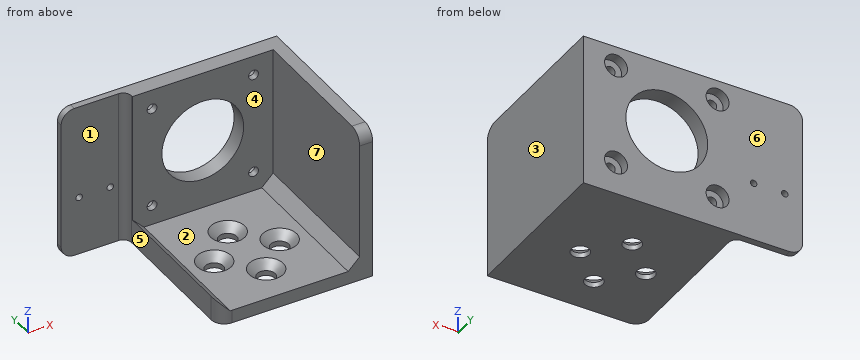
from build123d import *

# Parameters (mm, degrees)
SKETCH_2_W                  = 47
SKETCH_2_H                  = 47
EXTRUDE_1_DEPTH             = 4
SKETCH_3_W                  = 47
SKETCH_3_H                  = 2
EXTRUDE_2_DEPTH             = 43
SKETCH_4_W                  = 4
SKETCH_4_H                  = 45
EXTRUDE_3_DEPTH             = 43
SKETCH_5_R                  = 12.5
CUT_EXTRUDE_1_DEPTH         = 81.268300094
M3X0_5_2_D                  = 3
HOLE_WIZARD_M5_1_AT_2_COUNT = 2
HOLE_WIZARD_M5_1_AT_2_PITCH = 14.142135624
HOLE_WIZARD_M5_1_AT_3_COUNT = 2
HOLE_WIZARD_M5_1_AT_3_PITCH = 20
HOLE_WIZARD_M5_1_AT_4_COUNT = 2
HOLE_WIZARD_M5_1_AT_4_PITCH = 14.142135624
EXTRUDE_6_DEPTH             = 45
EXTRUDE_7_DEPTH             = 45
SKETCH_23_W                 = 67
SKETCH_23_H                 = 47
SKETCH_23_R                 = 3.5
SKETCH_23_R_2               = 12.5
EXTRUDE_10_DEPTH            = 3
M2X0_4_1_D                  = 2
SKETCH_27_W                 = 47
SKETCH_27_H                 = 1
CUT_EXTRUDE_2_DEPTH         = 20
FILLET_1_R                  = 2.5
FILLET_2_R                  = 4


with BuildPart() as part:
    # ｽｹｯﾁ2 → ﾎﾞｽ - 押し出し1 (new body)
    with BuildSketch(Plane.XY):
        with Locations((23.5, 23.5)):
            Rectangle(SKETCH_2_W, SKETCH_2_H)
    extrude(amount=EXTRUDE_1_DEPTH)

    # ｽｹｯﾁ3 → ﾎﾞｽ - 押し出し2 (add)
    with BuildSketch(Plane.XY.offset(4)):
        with Locations((23.5, 46)):
            Rectangle(SKETCH_3_W, SKETCH_3_H)
    extrude(amount=EXTRUDE_2_DEPTH)

    # ｽｹｯﾁ4 → ﾎﾞｽ - 押し出し3 (add)
    with BuildSketch(Plane.XY.offset(4)):
        with Locations((45, 22.5)):
            Rectangle(SKETCH_4_W, SKETCH_4_H)
    extrude(amount=EXTRUDE_3_DEPTH)

    # ｽｹｯﾁ5 → ｶｯﾄ - 押し出し1 (cut, through all)
    with BuildSketch(Plane.XZ.offset(-45)):
        with Locations(Location((21.5, 25.5, 0), (0, 0, 270))):
            Circle(SKETCH_5_R)
    extrude(amount=-CUT_EXTRUDE_1_DEPTH, mode=Mode.SUBTRACT)

    # M3x0.5 ねじ穴2 (through all)
    with Locations(Plane(origin=(0, 47, 0), x_dir=(1, 0, 0), z_dir=(0, 1, 0))):
        with Locations((6, -10), (37, -10), (37, -41), (6, -41)):
            Hole(M3X0_5_2_D / 2)

    # ｽｹｯﾁ14 → M5 平皿頭ねじ用皿穴1 (revolve, cut)
    with BuildSketch(Plane(origin=(11.5, 22, 4), x_dir=(0, -1, 0), z_dir=(1, 0, 0))):
        Polygon((0, 0), (0, 4), (2.75, 4), (2.75, 2.45), (5.2, 0), align=None)
    hole_wizard_m5_1 = revolve(axis=Axis((11.5, 22, 10.35), (0, 0, -1)), mode=Mode.SUBTRACT)

    # M5 平皿頭ねじ用皿穴1 at 2: M5 平皿頭ねじ用皿穴1 ×2
    with Locations(*[Vector(0.7071067811865475, 0.7071067811865476, 0) * (i * HOLE_WIZARD_M5_1_AT_2_PITCH) for i in range(1, HOLE_WIZARD_M5_1_AT_2_COUNT)]):
        add(hole_wizard_m5_1, mode=Mode.SUBTRACT)

    # M5 平皿頭ねじ用皿穴1 at 3: M5 平皿頭ねじ用皿穴1 ×2
    with Locations(*[(i * HOLE_WIZARD_M5_1_AT_3_PITCH, 0, 0) for i in range(1, HOLE_WIZARD_M5_1_AT_3_COUNT)]):
        add(hole_wizard_m5_1, mode=Mode.SUBTRACT)

    # M5 平皿頭ねじ用皿穴1 at 4: M5 平皿頭ねじ用皿穴1 ×2
    with Locations(*[Vector(0.7071067811865474, -0.7071067811865478, 0) * (i * HOLE_WIZARD_M5_1_AT_4_PITCH) for i in range(1, HOLE_WIZARD_M5_1_AT_4_COUNT)]):
        add(hole_wizard_m5_1, mode=Mode.SUBTRACT)

    # ｽｹｯﾁ17 → ﾎﾞｽ - 押し出し6 (add)
    with BuildSketch(Plane.XZ.offset(-45)):
        Polygon((43, 4), (39.5, 4), (43, 7.5), align=None)
    extrude(amount=EXTRUDE_6_DEPTH)

    # ｽｹｯﾁ19 → ﾎﾞｽ - 押し出し7 (add)
    with BuildSketch(Plane.XZ.offset(-45)):
        Polygon((0, 4), (3.5, 4), (0, 7.5), align=None)
    extrude(amount=EXTRUDE_7_DEPTH)

    # ｽｹｯﾁ23 → ﾎﾞｽ - 押し出し10 (add)
    with BuildSketch(Plane(origin=(0, 47, 0), x_dir=(1, 0, 0), z_dir=(0, 1, 0))):
        with Locations((13.5, -23.5)):
            Rectangle(SKETCH_23_W, SKETCH_23_H)
        with Locations(Location((6, -10, 0), (0, 0, 270))):
            Circle(SKETCH_23_R, mode=Mode.SUBTRACT)
        with Locations(Location((6, -41, 0), (0, 0, 270))):
            Circle(SKETCH_23_R, mode=Mode.SUBTRACT)
        with Locations(Location((37, -10, 0), (0, 0, 270))):
            Circle(SKETCH_23_R, mode=Mode.SUBTRACT)
        with Locations(Location((37, -41, 0), (0, 0, 270))):
            Circle(SKETCH_23_R, mode=Mode.SUBTRACT)
        with Locations(Location((21.5, -25.5, 0), (0, 0, 90))):
            Circle(SKETCH_23_R_2, mode=Mode.SUBTRACT)
    extrude(amount=EXTRUDE_10_DEPTH)

    # M2x0.4 ねじ穴1 (through all)
    with Locations(Plane(origin=(0, 50, 0), x_dir=(1, 0, 0), z_dir=(0, 1, 0))):
        with Locations((-5, -18), (-14.5, -18)):
            Hole(M2X0_4_1_D / 2)

    # ｽｹｯﾁ27 → ｶｯﾄ - 押し出し2 (cut)
    with BuildSketch(Plane.ZY.offset(20)):
        with Locations((23.5, 47.5)):
            Rectangle(SKETCH_27_W, SKETCH_27_H)
    extrude(amount=-CUT_EXTRUDE_2_DEPTH, mode=Mode.SUBTRACT)

    # ﾌｨﾚｯﾄ1
    fillet_1_edges = [part.edges().sort_by_distance(p)[0] for p in [
        (0, 48, 23.5),
    ]]
    fillet(fillet_1_edges, radius=FILLET_1_R)

    # ﾌｨﾚｯﾄ2
    fillet_2_edges = [part.edges().sort_by_distance(p)[0] for p in [
        (-20, 49, 47),
        (-20, 49, 0),
        (0, 0, 3.75),
        (45, 0, 47),
    ]]
    fillet(fillet_2_edges, radius=FILLET_2_R)


solid = part.part
The model under review builds one solid part; all positions refer to its coordinate system, in mm. Face numbers are marked on the shaded views. A direction names the side the tool comes from. Round coordinates to 2 decimals unless told otherwise and drop trailing zeros. Loops run counter-clockwise (first coordinate to the right, second up) from the corner with the lowest first, then second, coordinate; pieces in that order, holes last. Notation, with made-up numbers: (55, 43) -> (100, 43) arc R31 cw to (100, 70) -> close; hole circle Ø4 at (-0.75, 37). An arc over 180 degrees is marked (long way). Return JSON: item names as keys, results as strings.
(1) Add section C-C on z = 29. Write out the cut boundary in (x, y).
Solved:
{"outline": "(-20, 48) -> (-2.5, 48) arc R2.5 cw to (0, 45.5) -> (0, 45) -> (9.5, 45) -> (9.5, 50) -> (-20, 50) -> close; (33.5, 45) -> (43, 45) -> (43, 0) -> (47, 0) -> (47, 50) -> (33.5, 50) -> close"}
(2) For line 1 (X direction, y = 45.7, z = 41); line 2 (X direction, y = 49, z = 10); line 3 (X direction, y = 49.15, z = 18), list the stretches that pass through material, from the lowest coordinate up.
Solved:
{"line 1": "-0.01 to 4.5, 7.5 to 35.5, 38.5 to 47", "line 2": "-20 to 2.5, 9.5 to 33.5, 40.5 to 47", "line 3": "-20 to -15.5, -13.5 to -6, -4 to 11.5, 31.5 to 47"}
(3) For pin 1 (5 mm diameter, centred on x = -10.5, z = 14, fed in from -Y); pin 2 (1.8 mm diameter, centred on x = 6, z = 10, fed in from -Y); pin 3 (8 mm diameter, centred on x = 8, z = 38, fed in from -Y); pin 4 (3.5 mm diameter, centred on x = 37, z = 10, fed in from +Y), all flat-tipped, find the tip position at first contact; note any pin that passes through.
Solved:
{"pin 1": "y = 48", "pin 2": "through", "pin 3": "y = 45", "pin 4": "y = 47"}
(4) Add section D-D on y = 12. Write out the cut boundary in (x, z).
Solved:
{"outline": "(0, 0) -> (18.75, 0) -> (18.75, 1.55) -> (16.3, 4) -> (3.5, 4) -> (0, 7.5) -> close; (24.25, 0) -> (47, 0) -> (47, 47) -> (43, 47) -> (43, 7.5) -> (39.5, 4) -> (26.7, 4) -> (24.25, 1.55) -> close"}
(5) Add section A-A on y = 22. Write out the cut boundary in (x, z).
Solved:
{"outline": "(0, 0) -> (8.75, 0) -> (8.75, 1.55) -> (6.3, 4) -> (3.5, 4) -> (0, 7.5) -> close; (14.25, 0) -> (28.75, 0) -> (28.75, 1.55) -> (26.3, 4) -> (16.7, 4) -> (14.25, 1.55) -> close; (34.25, 0) -> (47, 0) -> (47, 47) -> (43, 47) -> (43, 7.5) -> (39.5, 4) -> (36.7, 4) -> (34.25, 1.55) -> close"}
(6) The part is to be moulded in two halves that separate along X. For the marked faces 1, 2 and 3, say which applies: released by +X, released by -X, zero draft, split by the parting line, or undercut.
Solved:
{"face 1": "zero draft", "face 2": "undercut", "face 3": "released by +X"}
(7) For the marked faces 4, 5, 6 and 7, list the 3-axis set-ups (+Z, -Z, +X, -X, +Y, -Y) from which the entire face can be reached by the end or side of a thin tool; tool diameter is ignored.
Solved:
{"face 4": "+Z, -Y", "face 5": "+Z, -Z, -X, -Y", "face 6": "+Z, -Z, +X, -X, +Y", "face 7": "+Z, -X, -Y"}
(8) Add section B-B on x = -5. Write out the cut boundary in (y, z), plus the area to 3 significant figures.
Solved:
{"outline": "(48, 0) -> (50, 0) -> (50, 17) -> (48, 17) -> close; (48, 19) -> (50, 19) -> (50, 47) -> (48, 47) -> close", "area": "90.0 mm2"}
